Check sheet for the drawn part. Datum: minimum x, y, z corner. Units: mm. A direction names the side the tool comes from. Give positions to 0.01 mm unless a question says otherwise; leave off trailing zeros. Order: outer loops, then holes, each group sorted by start corner. A loop starts at its lowest first (then second) coordinate and runs counter-clockwise, first axis right, second up. Notation, with made-up numbers: (86, 85.25) -> (116, 85.25) arc R17 cw to (116, 105.25) -> close; hole circle Ø9 at (56, 49.5). An arc over 180 degrees is marked (long way). Answer in a Markdown table with one row per item. Add a question column.
(1) Cross-section at B-B (y = 12.25). Record the cut outline in (x, z), then the cut area to 3 significant figures.
(2) Go/stop test with flat-tipped pins: pin 1 (5 mm diameter, centred on y = 23.5, z = 9.5, fed in from -X); pin 2 (6 mm diameter, centred on x = 7, z = 15, fed in from -Y). Record where each tip stops, or that it passes through.
(3) Cross-section at C-C (x = 10). Record the cut outline in (y, z).
(4) Cross-section at D-D (x = 46.5). Record the cut outline in (y, z), then the cut area to 3 significant figures.
(5) Set-up check for the marked faces 1, 2 and 3: record each of +Z, -Z, +X, -X, +Y, -Y from which the full face is reachable in a straight line by a thin tool's end or side.
(6) Cross-section at A-A (z = 31). Record the cut outline in (x, y).
(7) Thickness scan on L1, parallel to Y at x = 3, z = 23; L2, parallel to X at y = 5, z = 19; L3, parallel to Z at x = 44, y = 19.75. Record the ranges inside material, lowest first. Write a range as [from, to].
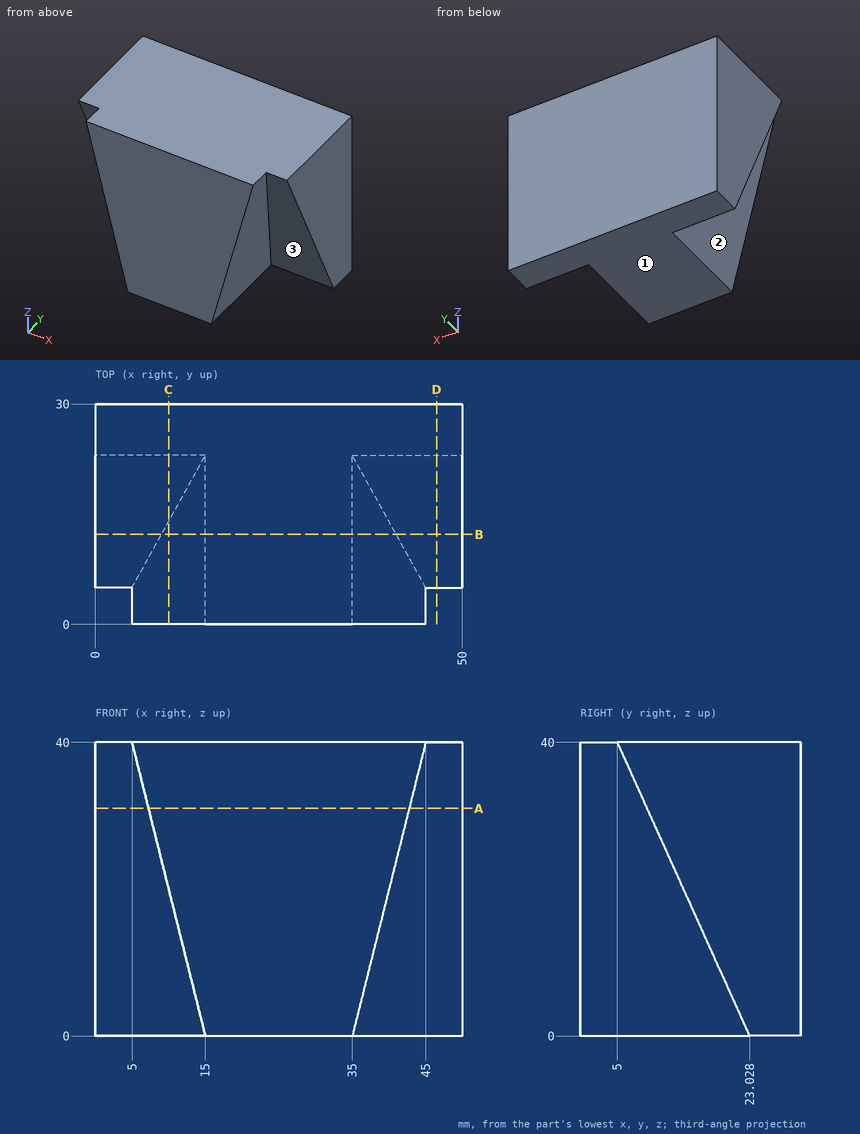
Answer below:
| question | item | result |
|---|---|---|
| 1 | outline | (0, 23.91) -> (9.02, 23.91) -> (15, 0) -> (35, 0) -> (40.98, 23.91) -> (50, 23.91) -> (50, 40) -> (0, 40) -> close |
| 1 | area | 1,430 mm² |
| 2 | pin 1 | stops at x = 0 |
| 2 | pin 2 | stops at y = 14.92 |
| 3 | outline | (0, 20) -> (14.01, 20) -> (23.03, 0) -> (30, 0) -> (30, 40) -> (0, 40) -> close |
| 4 | outline | (5, 40) -> (23.03, 0) -> (30, 0) -> (30, 40) -> close |
| 4 | area | 639 mm² |
| 5 | face 1 | -Z, +X, -X, +Y, -Y |
| 5 | face 2 | -Z, -X, -Y |
| 5 | face 3 | -Z, +X, -Y |
| 6 | outline | (0, 9.06) -> (7.25, 9.06) -> (7.25, 0) -> (42.75, 0) -> (42.75, 9.06) -> (50, 9.06) -> (50, 30) -> (0, 30) -> close |
| 7 | L1 | y = [12.66, 30] |
| 7 | L2 | x = [10.25, 39.75] |
| 7 | L3 | z = [7.27, 40] |
